Source: CAD feature listing. Evaluate the final solid. Frame: model axes, mm. Face numbers are marked on the shaded views. A direction names the side the tool comes from. Give positions to 0.01 mm unless a question says otherwise; leave off trailing zeros. Write each loop counter-clockwise with the first axis right and the second up, starting at its lowest first coordinate (ties: lowest second). Pieces come first, ordered by that corner, then holes. Notation, with made-up numbers: (87, 15) -> (101, 15) arc R17 ccw to (101, 20) -> close; hole circle Ø2 at (-28.75, 80). An arc over 180 degrees is marked (long way). Write item = value, one per line.
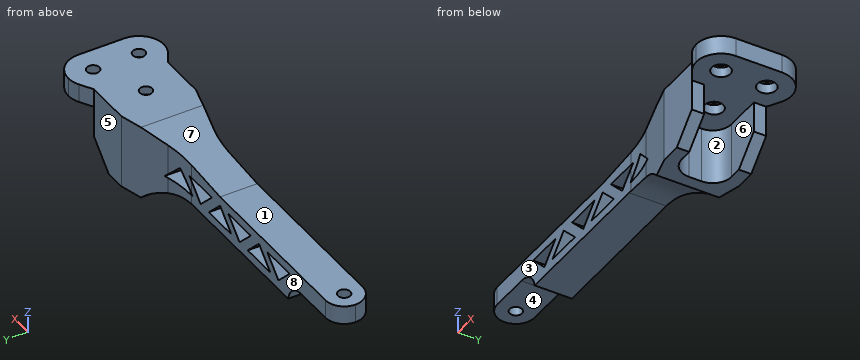
from build123d import *

# Parameters (mm, degrees)
BOSS_EXTRUDE1_DEPTH     = 77
SKETCH2_W               = 126.439286786
SKETCH2_H               = 23.5
CUT_EXTRUDE1_DEPTH      = 23.5
CUT_EXTRUDE1_DEPTH_BACK = 38.5
CUT_EXTRUDE2_DEPTH      = 23.5000001
CUT_EXTRUDE2_DEPTH_BACK = 22.5
SKETCH3_R               = 5
CUT_EXTRUDE3_DEPTH      = 46.0000001
CUT_EXTRUDE3_DEPTH_BACK = 16
SKETCH4_R               = 7.5
SKETCH4_R_2             = 5
CUT_EXTRUDE4_DEPTH      = 8


with BuildPart() as part:
    # Sketch1 → Boss-Extrude1 (new body)
    with BuildSketch(Plane(origin=(0, 0, 0), x_dir=(1, 0, 0), z_dir=(0, 1, 0))):
        with BuildLine():
            Line((0, 0), (126.439286786, 0))
            ThreePointArc((126.439286786, 0), (155.486661882, 5.85341657), (180, 22.5))
            Line((180, 22.5), (215, 22.5))
            Line((215, 22.5), (235, 2.5))
            Line((235, 2.5), (235, -22.5))
            Line((235, -22.5), (275, -22.5))
            Line((275, -22.5), (275, -37.5))
            Line((275, -37.5), (180, -37.5))
            Line((180, -37.5), (91, -30))
            Line((91, -30), (-65, -30))
            Line((-65, -30), (-65, -15))
            Line((-65, -15), (-17.748239349, -15))
            ThreePointArc((-17.748239349, -15), (-6.129289311, -10.747727085), (0, 0))
        make_face()
        Polygon((-2, -22.5), (13, -7.5), (28, -22.5), align=None, mode=Mode.SUBTRACT)
        Polygon((50, -22.5), (65, -7.5), (80, -22.5), align=None, mode=Mode.SUBTRACT)
        Polygon((54, -7.5), (39, -22.5), (24, -7.5), align=None, mode=Mode.SUBTRACT)
        Polygon((106, -7.5), (91, -22.5), (76, -7.5), align=None, mode=Mode.SUBTRACT)
        Polygon((158, -7.5), (143, -22.5), (128, -7.5), align=None, mode=Mode.SUBTRACT)
        Polygon((102, -22.5), (117, -7.5), (132, -22.5), align=None, mode=Mode.SUBTRACT)
    extrude(amount=BOSS_EXTRUDE1_DEPTH)

    # Sketch2 → Cut-Extrude1 (cut, two sides)
    with BuildSketch(Plane(origin=(0, 0, 0), x_dir=(-1, 0, 0), z_dir=(0, 0, -1))) as cut_extrude1_sk:
        with Locations((-63.219643393, 11.75)):
            Rectangle(SKETCH2_W, SKETCH2_H)
        with BuildLine():
            Line((50, 23.5), (0, 23.5))
            Line((0, 23.5), (0, 0))
            Line((0, 0), (65, 0))
            Line((65, 0), (65, 38.5))
            ThreePointArc((65, 38.5), (60.606601718, 27.893398282), (50, 23.5))
        make_face()
        with BuildLine():
            Line((0, 77), (0, 53.5))
            Line((0, 53.5), (50, 53.5))
            ThreePointArc((50, 53.5), (60.606601718, 49.106601718), (65, 38.5))
            Line((65, 38.5), (65, 77))
            Line((65, 77), (0, 77))
        make_face()
        with Locations((-63.219643393, 65.25)):
            Rectangle(SKETCH2_W, SKETCH2_H)
        with BuildLine():
            ThreePointArc((-154.88190451, 56.907417371), (-142.052619222, 54.355513863), (-129, 53.5))
            Line((-129, 53.5), (-126.439286786, 53.5))
            Line((-126.439286786, 53.5), (-126.439286786, 77))
            Line((-126.439286786, 77), (-255, 77))
            ThreePointArc((-255, 77), (-249.789539733, 76.309352755), (-244.938938469, 74.28511038))
            Line((-244.938938469, 74.28511038), (-235, 68.5))
            Line((-235, 68.5), (-198.146011872, 68.5))
            Line((-198.146011872, 68.5), (-154.88190451, 56.907417371))
        make_face()
        with BuildLine():
            ThreePointArc((-129, 23.5), (-142.052619222, 22.644486137), (-154.88190451, 20.092582629))
            Line((-154.88190451, 20.092582629), (-198.146011872, 8.5))
            Line((-198.146011872, 8.5), (-235, 8.5))
            Line((-235, 8.5), (-244.938938469, 2.71488962))
            ThreePointArc((-244.938938469, 2.71488962), (-249.789539733, 0.690647245), (-255, 0))
            Line((-255, 0), (-126.439286786, 0))
            Line((-126.439286786, 0), (-126.439286786, 23.5))
            Line((-126.439286786, 23.5), (-129, 23.5))
        make_face()
        with BuildLine():
            Line((-275, 0), (-255, 0))
            ThreePointArc((-255, 0), (-269.142135624, 5.857864376), (-275, 20))
            Line((-275, 20), (-275, 0))
        make_face()
        with BuildLine():
            ThreePointArc((-275, 57), (-269.142135624, 71.142135624), (-255, 77))
            Line((-255, 77), (-275, 77))
            Line((-275, 77), (-275, 57))
        make_face()
    extrude(amount=CUT_EXTRUDE1_DEPTH, mode=Mode.SUBTRACT)
    extrude(cut_extrude1_sk.sketch, amount=-CUT_EXTRUDE1_DEPTH_BACK, mode=Mode.SUBTRACT)

    # Sketch2<3> → Cut-Extrude2 (cut, two sides)
    with BuildSketch(Plane(origin=(0, 0, 0), x_dir=(-1, 0, 0), z_dir=(0, 0, -1))) as cut_extrude2_sk:
        with BuildLine():
            Line((-244.938938469, 2.71488962), (-235, 8.5))
            Line((-235, 8.5), (-235, 18.5))
            Line((-235, 18.5), (-205, 18.5))
            ThreePointArc((-205, 18.5), (-194.393398282, 22.893398282), (-190, 33.5))
            Line((-190, 33.5), (-190, 43.5))
            ThreePointArc((-190, 43.5), (-194.393398282, 54.106601718), (-205, 58.5))
            Line((-205, 58.5), (-235, 58.5))
            Line((-235, 58.5), (-235, 68.5))
            Line((-235, 68.5), (-244.938938469, 74.28511038))
            ThreePointArc((-244.938938469, 74.28511038), (-237.661873939, 66.969422485), (-235, 57))
            Line((-235, 57), (-235, 20))
            ThreePointArc((-235, 20), (-237.661873939, 10.030577515), (-244.938938469, 2.71488962))
        make_face()
    extrude(amount=CUT_EXTRUDE2_DEPTH, mode=Mode.SUBTRACT)
    extrude(cut_extrude2_sk.sketch, amount=-CUT_EXTRUDE2_DEPTH_BACK, mode=Mode.SUBTRACT)

    # Sketch3 → Cut-Extrude3 (cut, two sides)
    with BuildSketch(Plane(origin=(0, 0, 22.5), x_dir=(-1, 0, 0), z_dir=(0, 0, -1))) as cut_extrude3_sk:
        with Locations((-215, 38.5)):
            Circle(SKETCH3_R)
        with Locations((-255, 20.04)):
            Circle(SKETCH3_R)
        with Locations((-255, 56.96)):
            Circle(SKETCH3_R)
        with Locations((50, 38.5)):
            Circle(SKETCH3_R)
    extrude(amount=CUT_EXTRUDE3_DEPTH, mode=Mode.SUBTRACT)
    extrude(cut_extrude3_sk.sketch, amount=-CUT_EXTRUDE3_DEPTH_BACK, mode=Mode.SUBTRACT)

    # Sketch4 → Cut-Extrude4 (cut)
    with BuildSketch(Plane(origin=(0, 0, 22.5), x_dir=(-1, 0, 0), z_dir=(0, 0, -1))):
        with Locations((-215, 38.5)):
            Circle(SKETCH4_R)
        with Locations((-215, 38.5)):
            Circle(SKETCH4_R_2, mode=Mode.SUBTRACT)
        with Locations((-255, 20.04)):
            Circle(SKETCH4_R)
        with Locations((-255, 20.04)):
            Circle(SKETCH4_R_2, mode=Mode.SUBTRACT)
        with Locations((-255, 56.96)):
            Circle(SKETCH4_R)
        with Locations((-255, 56.96)):
            Circle(SKETCH4_R_2, mode=Mode.SUBTRACT)
    extrude(amount=-CUT_EXTRUDE4_DEPTH, mode=Mode.SUBTRACT)


solid = part.part
(1) Pull-direction query (Y, two-part tool) for the marked faces 6, 7 and 8; classes: pulls with the +Y half, pulls with the -Y half, needs draft (parallel to the pull), parting line crosses it, or undercut.
Values follow:
face_6 = undercut
face_7 = needs draft
face_8 = pulls with the +Y half
(2) Material intervals for line 1 (Y direction, x = 255, z = 25); line 2 (Y direction, x = 255, z = 33.75); line 3 (Y direction, x = 215, z = 25.75), sorted ascending.
Values follow:
line_1 = 0 to 12.54, 27.54 to 49.46, 64.46 to 77
line_2 = 0 to 15.04, 25.04 to 51.96, 61.96 to 77
line_3 = 8.5 to 31, 46 to 68.5
(3) Access query for the marked faces 1, 2, 3, 4 and 5. Directions: +Z, -Z, +X, -X, +Y, -Y. A direction counts if a zero-diameter tool reaches every point of the face in a straight line with its end or side. Return the directions, or none.
Values follow:
face_1 = +Z, -X, +Y, -Y
face_2 = -Z, +X
face_3 = +Z, -Z, -X, -Y
face_4 = -Z, -X, +Y, -Y
face_5 = +Z, -Z, -X, +Y
(4) Section query B-B (x = -30). Return loops of the section in (y, z).
Values follow:
outline = (23.5, 15) -> (53.5, 15) -> (53.5, 30) -> (23.5, 30) -> close
(5) Section query A-A (x = 96). Return loops of the section in (y, z).
Values follow:
outline = (23.5, 0) -> (53.5, 0) -> (53.5, 7.5) -> (23.5, 7.5) -> close; (23.5, 17.5) -> (53.5, 17.5) -> (53.5, 30.42) -> (23.5, 30.42) -> close
(6) First-contact query: pin 1 (6 mm diameter, centred on y = 30, z = -8.5, fed in from -X); pin 2 (9 mm diameter, centred on x = 42.5, y = 41, fed in from +Z); pin 3 (2 mm diameter, centred on x = 138, z = 8, fed in from -Y); pin 4 (13.5 mm diameter, centred on x = 255, y = 20.04, fed in from +Z). Flat tips, straight axial feed; report the tip coordinate or a pass-through.
Values follow:
pin_1 = 154.63
pin_2 = 30
pin_3 = 23.01
pin_4 = 37.5
